Geometry: final body of the model. Coordinates: model frame, mm. Give positions to 0.01 mm unless a question says otherwise; leave off trailing zeros. Loops run counter-clockwise (first coordinate to the right, second up) from the corner with the lowest first, then second, coordinate; pieces in that order, holes last. Notation, with made-up numbers: (72.25, -23.75) - (113.25, -23.75) arc R16 ccw to (113.25, 6.25) - close; hole circle Ø4 at (69, -19.5). An arc over 180 degrees is marked (long way). Answer in a Markdown table with one row per item.
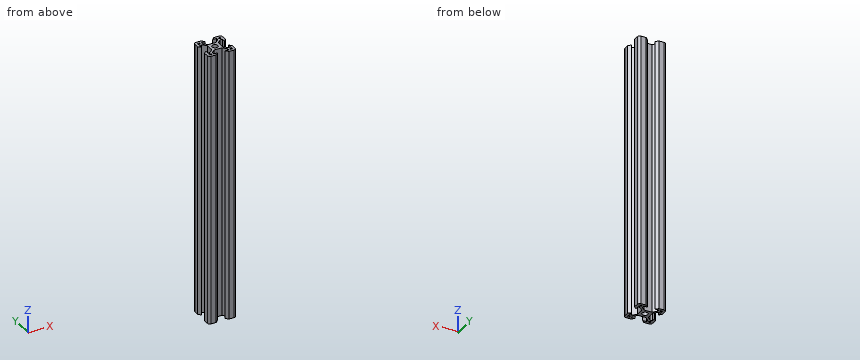
Autodesk Inventor part; units mm, degrees
ref_plane "Start Plane" through (0, 0, 80) normal (0, 0, 1) x (1, 0, 0)
ref_plane "End Plane" through (0, 0, 275) normal (0, 0, 1) x (1, 0, 0)
ref_plane "Work Plane5" through (475, -8, 80) normal (0, 0, -1) x (-1, 0, 0)
ref_plane "Start Plane" through (0, 0, 80) normal (0, 0, 1) x (1, 0, 0)
ref_plane "End Plane" through (0, 0, 275) normal (0, 0, 1) x (1, 0, 0)
sketch "Sketch" plane through (0, 0, 0) normal (0, 0, 1) x (1, 0, 0)
  line L0 (10, -4.5951) -> (10, -8.2)
  line L1 (-10, -8.2) -> (-10, -4.5951)
  line L2 (-10, 10) -> (10, -10) construction
  line L3 (10, 10) -> (-10, -10) construction
  circle A0 centre (0, 0) radius 2.1
  line L4 (-2.84, -3.9007) -> (2.84, -3.9007)
  line L5 (3.9007, -2.84) -> (3.9007, 2.84)
  line L6 (2.84, 3.9007) -> (-2.84, 3.9007)
  line L7 (-3.9007, 2.84) -> (-3.9007, -2.84)
  line L8 (-3.9007, -3.9007) -> (3.9007, 3.9007) construction
  line L9 (3.9007, -3.9007) -> (-3.9007, 3.9007) construction
  line L10 (-3.9007, -2.84) -> (-2.84, -3.9007) construction
  line L11 (-2.84, -3.9007) -> (-5.4993, -6.56)
  line L12 (-5.4993, -6.56) -> (-5.4993, -8.2)
  line L13 (-5.4993, -8.2) -> (-2.7951, -8.2)
  line L14 (-2.7951, -8.2) -> (-4.5951, -10)
  line L15 (0, 0) -> (0, -3.9007) construction
  line L16 (3.9007, -2.84) -> (2.84, -3.9007) construction
  line L17 (2.84, -3.9007) -> (5.4993, -6.56)
  line L18 (5.4993, -6.56) -> (5.4993, -8.2)
  line L19 (5.4993, -8.2) -> (2.7951, -8.2)
  line L20 (2.7951, -8.2) -> (4.5951, -10)
  line L21 (-2.84, -3.9007) -> (-3.9007, -2.84) construction
  line L22 (-3.9007, -2.84) -> (-6.56, -5.4993)
  line L23 (-6.56, -5.4993) -> (-8.2, -5.4993)
  line L24 (-8.2, -5.4993) -> (-8.2, -2.7951)
  line L25 (-8.2, -2.7951) -> (-10, -4.5951)
  line L26 (3.9007, -2.84) -> (6.56, -5.4993)
  line L27 (6.56, -5.4993) -> (8.2, -5.4993)
  line L28 (8.2, -5.4993) -> (8.2, -2.7951)
  line L29 (8.2, -2.7951) -> (10, -4.5951)
  arc A1 (-10, -8.2) -> (-8.2, -10) centre (-8.2, -8.2) ccw
  arc A2 (8.2, -10) -> (10, -8.2) centre (8.2, -8.2) ccw
  line L30 (-8.2, -6.56) -> (-7.7111, -6.56)
  line L31 (-6.6505, -8.2) -> (-8.2, -8.2)
  line L32 (-8.2, -8.2) -> (-8.2, -6.56)
  line L33 (-6.6505, -7.6207) -> (-7.7111, -6.56)
  line L34 (-6.6505, -7.6207) -> (-6.6505, -8.2)
  line L35 (8.2, -6.56) -> (7.7111, -6.56)
  line L36 (6.6505, -8.2) -> (8.2, -8.2)
  line L37 (8.2, -8.2) -> (8.2, -6.56)
  line L38 (6.6505, -7.6207) -> (7.7111, -6.56)
  line L39 (6.6505, -7.6207) -> (6.6505, -8.2)
  line L40 (8.2, -10) -> (4.5951, -10)
  line L41 (-4.5951, -10) -> (-8.2, -10)
  line L42 (-3.9007, 0) -> (3.9007, 0) construction
  line L43 (10, 4.5951) -> (10, 8.2)
  line L44 (-10, 8.2) -> (-10, 4.5951)
  line L45 (-2.84, 3.9007) -> (2.84, 3.9007)
  line L46 (-3.9007, 2.84) -> (-2.84, 3.9007) construction
  line L47 (-2.84, 3.9007) -> (-5.4993, 6.56)
  line L48 (-5.4993, 6.56) -> (-5.4993, 8.2)
  line L49 (-5.4993, 8.2) -> (-2.7951, 8.2)
  line L50 (-2.7951, 8.2) -> (-4.5951, 10)
  line L51 (2.84, 3.9007) -> (5.4993, 6.56)
  line L52 (5.4993, 6.56) -> (5.4993, 8.2)
  line L53 (5.4993, 8.2) -> (2.7951, 8.2)
  line L54 (2.7951, 8.2) -> (4.5951, 10)
  line L55 (3.9007, 2.84) -> (2.84, 3.9007) construction
  line L56 (-8.2, 2.7951) -> (-10, 4.5951)
  line L57 (-2.84, 3.9007) -> (-3.9007, 2.84) construction
  line L58 (-3.9007, 2.84) -> (-6.56, 5.4993)
  line L59 (-6.56, 5.4993) -> (-8.2, 5.4993)
  line L60 (-8.2, 5.4993) -> (-8.2, 2.7951)
  line L61 (3.9007, 2.84) -> (6.56, 5.4993)
  line L62 (6.56, 5.4993) -> (8.2, 5.4993)
  line L63 (8.2, 5.4993) -> (8.2, 2.7951)
  line L64 (8.2, 2.7951) -> (10, 4.5951)
  arc A3 (-8.2, 10) -> (-10, 8.2) centre (-8.2, 8.2) ccw
  arc A4 (10, 8.2) -> (8.2, 10) centre (8.2, 8.2) ccw
  line L65 (-8.2, 6.56) -> (-7.7111, 6.56)
  line L66 (-6.6505, 8.2) -> (-8.2, 8.2)
  line L67 (-8.2, 8.2) -> (-8.2, 6.56)
  line L68 (-6.6505, 7.6207) -> (-7.7111, 6.56)
  line L69 (-6.6505, 7.6207) -> (-6.6505, 8.2)
  line L70 (8.2, 6.56) -> (7.7111, 6.56)
  line L71 (6.6505, 7.6207) -> (7.7111, 6.56)
  line L72 (8.2, 8.2) -> (8.2, 6.56)
  line L73 (6.6505, 7.6207) -> (6.6505, 8.2)
  line L74 (6.6505, 8.2) -> (8.2, 8.2)
  line L75 (8.2, 10) -> (4.5951, 10)
  line L76 (-4.5951, 10) -> (-8.2, 10)
  line L77 (-8.2, 10) -> (-4.5951, 10)
  line L78 (4.5951, 10) -> (8.2, 10)
  point P0 (8.2, -8.2)
  point P1 (0, 3.9007)
  point P2 (8.2, 8.2)
  dimension "Width" = 20
  dimension "Height" = 20
  dimension "d2" = 4.2
  dimension "d3" = 1.5
  dimension "d4" = 1.64
  dimension "d6" = 5.68
  dimension "d7" = 1.8
  dimension "d9" = 1.5
extrude "Body" add sketch "Sketch" along normal up to surface (195 mm away) from surface at 80
sketch "Sketch4" plane through (0, 0, 0) normal (0, 0, 1) x (1, 0, 0)
  line L0 (0, 0) -> (10, 0)
ref_plane "Work Plane4" through (0, 0, 0) normal (0, -1, 0) x (1, 0, 0)
sketch "Sketch5" plane through (0, 0, 0) normal (0, -1, 0) x (1, 0, 0)
  line L0 (-2, 80) -> (12, 80) construction
  line L1 (-2, 275) -> (12, 275) construction
  dimension "d17" = 195
ref_plane "Work Plane5" through (475, -8, 80) normal (0, 0, -1) x (-1, 0, 0)
split "Split1" plane through (475, -8, 80) removes the side toward (0, 0, -1)
equation "\"G_OFFSET_START\" = -80"
equation "\"G_OFFSET_END\" = 0"
equation "\"d12\" = -G_OFFSET_START"
equation "\"d13\" = Length + G_OFFSET_END"
equation "\"G_L\" = d17"
properties part number "V-slot 20 mm x 20 mm" material "Aluminum 6061"
Q1. Material intervals for line 1 along Y through (x, z) = (-8, 182); line 2 along Y through (x, z) = (-4.25, 89.5); line 3 along X through (y, z) = (-3.25, 242.5), sorted ascending.
Check values:
| item | result |
|---|---|
| line 1 | -10 to -8.2, -6.56 to -5.5, 5.5 to 6.56, 8.2 to 10 |
| line 2 | -9.65 to -8.2, -5.31 to -3.19, 3.19 to 5.31, 8.2 to 9.65 |
| line 3 | -8.65 to -8.2, -4.31 to 4.31, 8.2 to 8.65 |
Q2. Cut plane A-A (x = 0). Output: boundary loops of the cut face in (y, z), and give its area (3 significant figures).
Check values:
| item | result |
|---|---|
| outline | (-3.9, 80) - (-2.1, 80) - (-2.1, 275) - (-3.9, 275) - close; (2.1, 80) - (3.9, 80) - (3.9, 275) - (2.1, 275) - close |
| area | 702 mm² |
Q3. Cut plane C-C (z = 200). Give the number of separate pieces and of enclosed holes in the cut face, and give its area (3 significant figures).
Check values:
| item | result |
|---|---|
| separate pieces | 1 |
| enclosed holes | 5 |
| area | 161 mm² |
Q4. First-contact query: pin 1 (1 mm diameter, centred on y = -2.5, z = 123.5, fed in from +X); pin 2 (6 mm diameter, centred on x = -0.5, z = 160.5, fed in from +Y); pin 3 (3 mm diameter, centred on x = -2.5, z = 149, fed in from +Y). Flat tips, straight axial feed; report the tip coordinate or a pass-through.
Check values:
| item | result |
|---|---|
| pin 1 | x = 8.4 |
| pin 2 | y = 8.9 |
| pin 3 | y = 9.4 |
